Autodesk Inventor part; units mm, degrees
ref_plane "YZ Plane" through (0, 0, 0) normal (1, 0, 0) x (0, 1, 0)
ref_plane "XZ Plane" through (0, 0, 0) normal (0, 1, 0) x (-1, 0, 0)
ref_plane "XY Plane" through (0, 0, 0) normal (0, 0, 1) x (1, 0, 0)
sketch "Sketch1" plane through (0, 0, 0) normal (0, 0, 1) x (1, 0, 0)
  line L0 (3.6, 0) -> (3.6, 8)
  line L1 (-3.6, 8) -> (-3.6, 0)
  arc A0 (3.6, 8) -> (-3.6, 8) centre (0, 8) ccw
  circle A1 centre (0, 8) radius 2.4
  circle A2 centre (0, 8) radius 3.2
  circle A3 centre (0, 0) radius 3.2
  circle A4 centre (0, 0) radius 2.4
  line L2 (0, 0) -> (0, 8) construction
  line L3 (-2.8, 5.7373) -> (-2.8, 2.2627)
  line L4 (2.8, 5.7373) -> (2.8, 2.2627)
  arc A5 (-2.8, 5.7373) -> (2.8, 5.7373) centre (0, 8) ccw
  arc A6 (2.8, 2.2627) -> (-2.8, 2.2627) centre (0, 0) ccw
  arc A7 (-3.6, 0) -> (3.6, 0) centre (0, 0) ccw
  line L5 (0, 0) -> (0, -8) construction
  dimension "d8" = 4.8
  dimension "d9" = 6.4
  dimension "d32" = 7.2
  dimension "d34" = 8
  dimension "d36" = 0.8
extrude "Extrusion1" add sketch "Sketch1" along normal mid plane 8 contours A7 L1 A0 L0 | A2 | A3 | A5 L4 A6 L3
sketch "Sketch6" plane through (0, 0, 4) normal (0, 0, 1) x (1, 0, 0)
  circle A0 centre (0, 0) radius 2.4
  circle A1 centre (0, 8) radius 2.4
  circle A2 centre (0, 0) radius 3.2
  circle A3 centre (0, 8) radius 3.2
  arc A4 (2.8, 2.2627) -> (-2.8, 2.2627) centre (0, 0) ccw
  line L0 (-2.8, 5.7373) -> (-2.8, 2.2627)
  arc A5 (-2.8, 5.7373) -> (2.8, 5.7373) centre (0, 8) ccw
  line L1 (2.8, 5.7373) -> (2.8, 2.2627)
extrude "Extrusion7" cut sketch "Sketch6" against normal blind 0.8 contours A2 | A3
extrude "Extrusion8" cut sketch "Sketch6" against normal blind 3.1 contours A4 L0 A5 L1
mirror "Mirror1" about plane through (0, 0, 0) normal (0, 0, 1) of "Extrusion7", "Extrusion8"
fillet "Fillet1" radius 0.1 6 edges at (0, 11.6, 4) (3.6, 4, 4) (-3.6, 4, 4) (0, 11.6, -4) (-3.6, 4, -4) (3.6, 4, -4)
fillet "Fillet1" radius 0.4 8 edges at (-2.8, 2.2627, 2.45) (-2.8, 5.7373, 2.45) (2.8, 2.2627, 2.45) (2.8, 5.7373, 2.45) (2.8, 5.7373, -2.45) (2.8, 2.2627, -2.45) (-2.8, 2.2627, -2.45) (-2.8, 5.7373, -2.45)
equation "\"d8\" = tpd"
equation "\"d9\" = tsd"
equation "\"d32\" = tlad"
equation "\"d34\" = lu"
equation "\"d14\" = lu"
equation "\"d41\" = tsl"
equation "\"d45\" = lf"
equation "\"d46\" = tf"
properties part number "43857-LtBluishGray" material "ABS Plastic"
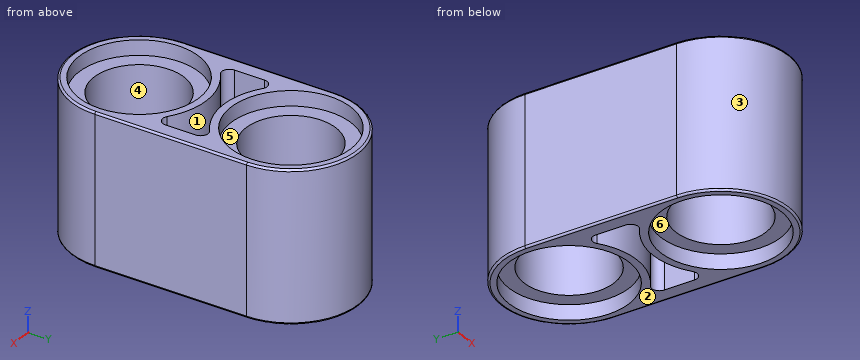
The listing builds one solid part. Answer for the finished solid, in the listing's coordinates (mm). Face numbers are marked on the shaded views. A direction names the side the tool comes from. Give positions to 0.01 mm unless a question says otherwise; leave off trailing zeros. Order: outer loops, then holes, each group sorted by start corner. A loop starts at its lowest first (then second) coordinate and runs counter-clockwise, first axis right, second up. Notation, with made-up numbers: M 2,54 L 27,54 A20 ccw 27,69 Z; hole C 3,21 d5. An arc over 180 degrees is marked long. Put each result on its own line as item: value. Start each with the question number.
Item 1: The part is cut by section C-C, the plane z = 0.25. Determine the outline of the cut face in (x, y).
Item 2: For a pull along Y with two mould halves and no side action, classify the marked faces 1, 2 and 3 as +Y half, -Y half, draft (parallel to the pull), parting line (faces both ways), or undercut.
Item 3: The part is cut by section D-D, the plane x = 0. State how many separate pieces and enclosed holes the cut face has, and give its area (3 significant figures).
Item 4: Which of the six approach directions +Z, -Z, +X, -X, +Y, -Y give full straight-line access (tool end or side, diameter ignored) to the marked faces 4, 5 and 6?
Item 5: The part is cut by section B-B, the plane y = 0.75. Determine the outline of the cut face in (x, z).
Item 6: Flat-ended cylindrical pins translate along their axes: P1, Ø2, axis at x = 3, z = 0, coming from the +Y side; P2, Ø1.9, axis at x = -1, y = 0.5, coming from the -Z side; P3, Ø3, axis at x = -2.5, z = 2.5, coming from the +Y side; P4, Ø3, axis at x = 1, y = 8.5, coming from the -Z side. Find the tip coordinate at first contact, or state that the pin passes through.
Item 7: Find the intervals of material crossed by line 1 along Y through (x, z) = (0, -0.75); line 2 along Y through (x, z) = (0, 3.6); line 3 along Y through (x, z) = (-0.5, 2.5), in increasing order.
Item 8: The part is cut by section A-A, the plane z = -1.5. Determine the outline of the cut face in (x, y), and give its area (3 significant figures).
Answer key:
1. outline: M -3.6,0 A3.6 ccw 3.6,0 L 3.6,8 A3.6 ccw -3.6,8 Z; hole C 0,0 d4.8; hole C 0,8 d4.8
2. face 1: undercut
2. face 2: draft
2. face 3: -Y half
3. separate pieces: 3
3. enclosed holes: 0
3. area: 34.7 mm²
4. face 4: +Z, -Z
4. face 5: +Z
4. face 6: -Z
5. outline: M -3.6,-3.9 A0.1 ccw -3.5,-4 L -3.11,-4 L -3.11,-3.2 L -2.28,-3.2 L -2.28,3.2 L -3.11,3.2 L -3.11,4 L -3.5,4 A0.1 ccw -3.6,3.9 Z; M 2.28,-3.2 L 3.11,-3.2 L 3.11,-4 L 3.5,-4 A0.1 ccw 3.6,-3.9 L 3.6,3.9 A0.1 ccw 3.5,4 L 3.11,4 L 3.11,3.2 L 2.28,3.2 Z
6. P1: stops at y = 10.99
6. P2: passes through
6. P3: stops at y = 11.46
6. P4: stops at z = -3.2
7. line 1: y = -3.6 to -2.4, 2.4 to 5.6, 10.4 to 11.6
7. line 2: y = -3.6 to -3.2, 3.2 to 3.6, 4.4 to 4.8, 11.2 to 11.6
7. line 3: y = -3.57 to -2.35, 2.35 to 3.57, 4.43 to 5.65, 10.35 to 11.57
8. outline: M -3.6,0 A3.6 ccw 3.6,0 L 3.6,8 A3.6 ccw -3.6,8 Z; hole M -2.8,3.2 A0.4 ccw -2.16,2.88 A3.6 cw 2.16,2.88 A0.4 ccw 2.8,3.2 L 2.8,4.8 A0.4 ccw 2.16,5.12 A3.6 cw -2.16,5.12 A0.4 ccw -2.8,4.8 Z; hole C 0,0 d4.8; hole C 0,8 d4.8
8. area: 53.8 mm²
